```python
from build123d import *

# Parameters (mm, degrees)
SKETCH_1_W               = 42
SKETCH_1_H               = 42
SKETCH_1_R               = 1.5
SKETCH_1_R_2             = 11.5
EXTRUDE_1_DEPTH          = 3
EXTRUDE_2_DEPTH          = 20
SKETCH_5_R               = 21.25
CUT_EXTRUDE_3_DEPTH      = 5
CUT_EXTRUDE_4_DEPTH      = 3
PATTERN_CIRCULAR_1_COUNT = 4


with BuildPart() as part:
    # 草图1 → 凸台-拉伸1 (new body)
    with BuildSketch(Plane.XY):
        Rectangle(SKETCH_1_W, SKETCH_1_H)
        with Locations((15.5, 15.5)):
            Circle(SKETCH_1_R, mode=Mode.SUBTRACT)
        with Locations((15.5, -15.5)):
            Circle(SKETCH_1_R, mode=Mode.SUBTRACT)
        with Locations((-15.5, -15.5)):
            Circle(SKETCH_1_R, mode=Mode.SUBTRACT)
        with Locations((-15.5, 15.5)):
            Circle(SKETCH_1_R, mode=Mode.SUBTRACT)
        Circle(SKETCH_1_R_2, mode=Mode.SUBTRACT)
    extrude(amount=EXTRUDE_1_DEPTH)

    # 草图2 → 凸台-拉伸2 (add)
    with BuildSketch(Plane(origin=(0, 0, 0), x_dir=(-1, 0, 0), z_dir=(0, 0, -1))):
        with BuildLine():
            Line((17.5, 14.142135624), (17.5, -14.142135624))
            ThreePointArc((17.5, -14.142135624), (22.5, 0), (17.5, 14.142135624))
        make_face()
        with BuildLine():
            ThreePointArc((-14.142135624, -17.5), (0, -22.5), (14.142135624, -17.5))
            Line((14.142135624, -17.5), (-14.142135624, -17.5))
        make_face()
        with BuildLine():
            Line((-14.142135624, 17.5), (14.142135624, 17.5))
            ThreePointArc((14.142135624, 17.5), (0, 22.5), (-14.142135624, 17.5))
        make_face()
        with BuildLine():
            ThreePointArc((-17.5, 14.142135624), (-22.5, 0), (-17.5, -14.142135624))
            Line((-17.5, -14.142135624), (-17.5, 14.142135624))
        make_face()
    extrude(amount=-EXTRUDE_2_DEPTH)

    # 草图5 → 切除-拉伸3 (cut)
    with BuildSketch(Plane.XY.offset(20)):
        Circle(SKETCH_5_R)
    extrude(amount=-CUT_EXTRUDE_3_DEPTH, mode=Mode.SUBTRACT)

    # 草图6 → 切除-拉伸4 (cut)
    with BuildSketch(Plane(origin=(0, 0, 0), x_dir=(-1, 0, 0), z_dir=(0, 0, -1))):
        Polygon((18.3, 17.116580754), (15.5, 18.733161507), (12.7, 17.116580754), (12.7, 13.883419246), (15.5, 12.266838493), (18.3, 13.883419246), align=None)
    cut_extrude_4 = extrude(amount=-CUT_EXTRUDE_4_DEPTH, mode=Mode.SUBTRACT)

    # 阵列(圆周)1: 切除-拉伸4 ×4 about axis
    pattern_circular_1_axis = Axis((0, 0, 0), (0, 0, 1))
    for i in range(1, PATTERN_CIRCULAR_1_COUNT):
        add(cut_extrude_4.rotate(pattern_circular_1_axis, i * 360 / PATTERN_CIRCULAR_1_COUNT), mode=Mode.SUBTRACT)


solid = part.part
```
Read the model definition and answer for the solid it produces. Units are mm, in the model's axes. A direction names the side the tool comes from. Give positions to 0.01 mm unless a question says otherwise; leave off trailing zeros. Loops run counter-clockwise (first coordinate to the right, second up) from the corner with the lowest first, then second, coordinate; pieces in that order, holes last.
Item 1: The part is cut by section B-B (z = 11.25). Write down the section's boundary in (x, y), and give its area (3 significant figures).
Item 2: Each of these flat-tipped pins is pushed along its axis until it touches: pin 1 Ø1 at (y, z) = (8.5, 6) entering from +X; pin 2 Ø10 at (x, z) = (8.5, 6.5) entering from +Y; pin 3 Ø4 at (x, y) = (4, 18.5) entering from +Z. Where does it stop, or does it pass through?
Item 3: The part is cut by section D-D (z = 17.25). Write down the section's boundary in (x, y), and give its area (3 significant figures).
Item 4: The mould has two halves that part along X. Classify faces 1 (the flat face through (13.086, 14.08, 1.479)), 2 (the flat face through (-19, 0, 15)), 3 (the flat face through (18, 18, 3)), 4 (the flat face through (-21, -15, 1)): released by +X, released by -X, zero draft, split by the parting line, or undercut.
Item 5: Find the intervals of material crossed by line 1 along Y through (x, z) = (0, 1.95); line 2 along Y through (x, z) = (0.5, 7.5); line 3 along X through (y, z) = (-19.5, 2), in increasing order.
Item 6: For faces 5 (the flat face through (16.92, -17.914, 1.479)), 6 (the flat face through (14.12, -17.936, 1.479)), 7 (the flat face through (14, -21, 1)), 8 (the cylindrical face through (-0.2, 22.5, 9.9)), determine the directions among +Z, -Z, +X, -X, +Y, -Y from which every point of the face is accessible in a straight line to the end or side of a thin tool.
Item 7: The part is cut by section A-A (x = 0). Write down the section's boundary in (y, z).
Taken from the geometry:
1. outline: (-17.5, -14.14) - (-17.5, 14.14) arc R22.5 ccw to start; (-14.14, -17.5) arc R22.5 ccw to (14.14, -17.5) - close; (-14.14, 17.5) - (14.14, 17.5) arc R22.5 ccw to start; (17.5, -14.14) arc R22.5 ccw to (17.5, 14.14) - close
1. area: 386 mm2
2. pin 1: stops at x = 21.03
2. pin 2: stops at y = 22.23
2. pin 3: stops at z = 15
3. outline: (-17.5, -14.14) - (-17.5, -12.05) arc R21.25 cw to (-17.5, 12.05) - (-17.5, 14.14) arc R22.5 ccw to start; (-14.14, -17.5) arc R22.5 ccw to (14.14, -17.5) - (12.05, -17.5) arc R21.25 cw to (-12.05, -17.5) - close; (-14.14, 17.5) - (-12.05, 17.5) arc R21.25 cw to (12.05, 17.5) - (14.14, 17.5) arc R22.5 ccw to start; (17.5, -14.14) arc R22.5 ccw to (17.5, 14.14) - (17.5, 12.05) arc R21.25 cw to (17.5, -12.05) - close
3. area: 141 mm2
4. face 1: undercut
4. face 2: undercut
4. face 3: zero draft
4. face 4: released by -X
5. line 1: y = -22.5 to -11.5, 11.5 to 22.5
5. line 2: y = -22.49 to -17.5, 17.5 to 22.49
5. line 3: x = -21 to 21
6. face 5: +Z, -Z
6. face 6: -Z
6. face 7: +Z, -Z, +X, -Y
6. face 8: +Z, +Y
7. outline: (-22.5, 0) - (-11.5, 0) - (-11.5, 3) - (-17.5, 3) - (-17.5, 15) - (-21.25, 15) - (-21.25, 20) - (-22.5, 20) - close; (11.5, 0) - (22.5, 0) - (22.5, 20) - (21.25, 20) - (21.25, 15) - (17.5, 15) - (17.5, 3) - (11.5, 3) - close
